```python
from build123d import *

# Parameters (mm, degrees)
F0_R     = 5.9507315311
F1_DEPTH = 2.5


with BuildPart() as f1:
    # F0 (on Top) → F1 (new body, symmetric)
    with BuildSketch(Plane.XY):
        Circle(F0_R)
        Polygon((1.5118795027, 3.65), (3.65, 1.5118795027), (3.65, -1.5118795027), (1.5118795027, -3.65), (-1.5118795027, -3.65), (-3.65, -1.5118795027), (-3.65, 1.5118795027), (-1.5118795027, 3.65), align=None, mode=Mode.SUBTRACT)
    extrude(amount=F1_DEPTH, both=True)


solid = f1.part
```
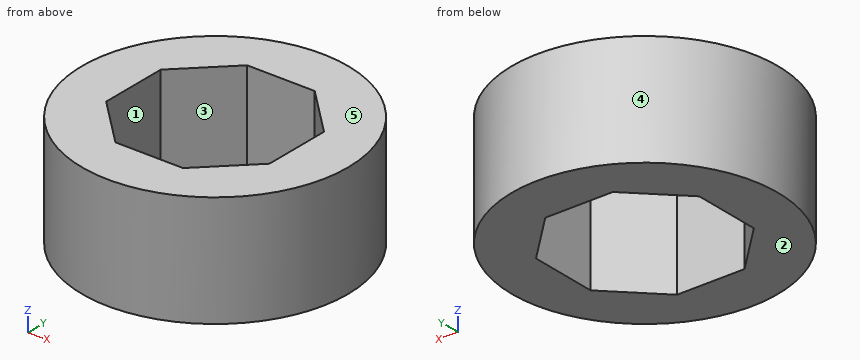
Model file for the job. Use its own axes, mm. Face numbers are marked on the shaded views. A direction names the side the tool comes from. Coordinates: 2 decimals unless noted, no trailing zeros. Order: outer loops, then holes, each group sorted by start corner. A loop starts at its lowest first (then second) coordinate and runs counter-clockwise, first axis right, second up. Notation, with made-up numbers: M 0.5,-13.75 L 51.5,-13.75 A9 ccw 51.5,-1.75 Z; hole C 25.5,77 d10. An arc over 180 degrees is marked long. Answer as CSV lines item,"result".
(1) Flat gauge pins, fed straight in: pin 1 (1.5 mm diameter, centred on y = 0.5, z = 1, fed in from -X); pin 2 (1 mm diameter, centred on y = 2.5, z = -2, fed in from -X); pin 3 (1 mm diameter, centred on x = 2.5, z = -1.5, fed in from -Y). Where does each tip first touch, or does it go through?
Geometry says:
pin 1,"stops at x = -5.95"
pin 2,"stops at x = -5.6"
pin 3,"stops at y = -5.6"
(2) Wall check: line 1 along Y through (x, z) = (0, 0.6); line 2 along Y through (x, z) = (2.5, 0.85); line 3 along X through (y, z) = (3.5, 2.1). Give the ranges that are in metal, low to high.
Geometry says:
line 1,"y = -5.95 to -3.65, 3.65 to 5.95"
line 2,"y = -5.4 to -2.66, 2.66 to 5.4"
line 3,"x = -4.81 to -1.66, 1.66 to 4.81"
(3) 3-axis set-ups, long thin cutter, end or side, ignore diameter. For the marked faces 1 and 2: which of +Z, -Z, +X, -X, +Y, -Y reach the whole face in a straight line?
Geometry says:
face 1,"+Z, -Z"
face 2,"-Z, +X, -X, +Y, -Y"
(4) Band-saw the part on B-B, the plane z = 0.75. List the corners of the cut face in (x, y).
Geometry says:
outline,"C 0,0 d11.9; hole M -3.65,-1.51 L -1.51,-3.65 L 1.51,-3.65 L 3.65,-1.51 L 3.65,1.51 L 1.51,3.65 L -1.51,3.65 L -3.65,1.51 Z"
(5) Band-saw the part on D-D, the plane y = -4.5. List the corners of the cut face in (x, z).
Geometry says:
outline,"M -3.89,-2.5 L 3.89,-2.5 L 3.89,2.5 L -3.89,2.5 Z"
(6) Band-saw the part on A-A, the plane x = 0. List the corners of the cut face in (y, z), then the cut area to 3 significant figures.
Geometry says:
outline,"M -5.95,-2.5 L -3.65,-2.5 L -3.65,2.5 L -5.95,2.5 Z; M 3.65,-2.5 L 5.95,-2.5 L 5.95,2.5 L 3.65,2.5 Z"
area,"23.0 mm2"
(7) Pull direction X, two halves, no side cores. Call the marked faces 3, 4 and 5: +X half, -X half, draft (parallel to the pull), parting line (faces both ways), or undercut.
Geometry says:
face 3,"undercut"
face 4,"parting line"
face 5,"draft"
